Verification items for this drawing (mm, ordinates from the low corner). A direction names the side the tool comes from. Coordinates: 2 decimals unless noted, no trailing zeros. Order: outer loops, then holes, each group sorted by start corner. A loop starts at its lowest first (then second) coordinate and runs counter-clockwise, first axis right, second up. Notation, with made-up numbers: M 56,-11 L 113,-11 A31 ccw 113,17 Z; hole C 51,-9.75 d7. An arc over 180 degrees is marked long. One line per item, written item: value. Start each with the question number.
1) Sectioned sample at C-C, the plane y = 11.5. Enter the section's corners in (x, z).
2) Sectioned sample at D-D, the plane z = 6.5. Enter the section's corners in (x, y).
3) Sectioned sample at A-A, the plane x = 25. Enter the section's corners in (y, z).
4) Draft check along X on the marked faces 1, 2, 3 and 4. Enter one of: pulls with the +X half, pulls with the -X half, needs draft (parallel to the pull), parting line crosses it, or undercut.
5) Access from +Z, -Z, +X, -X, +Y, -Y to the whole of each face (thin tool, end or side, straight path). Record for the marked faces 5 and 6.
6) Sectioned sample at B-B, the plane z = 21.5. Enter the section's corners in (x, y).
7) Thickness scan on L1, parallel to X at y = 19, z = 24.5; L2, parallel to Y at x = 31, z = 13. Record the ranges inside material, lowest first. Write a range as from..to.
8) Go/stop test with flat-tipped pins: P1, Ø12, axis at x = 25, y = 7.5, coming from the +Z side; P2, Ø1.5, axis at x = 10.5, z = 22.5, coming from the +Y side; P3, Ø13, axis at y = 25, z = 21.5, coming from the -X side; P4, Ø3, axis at y = 23.5, z = 24.5, coming from the +X side. Record where each tip stops, or that it passes through.
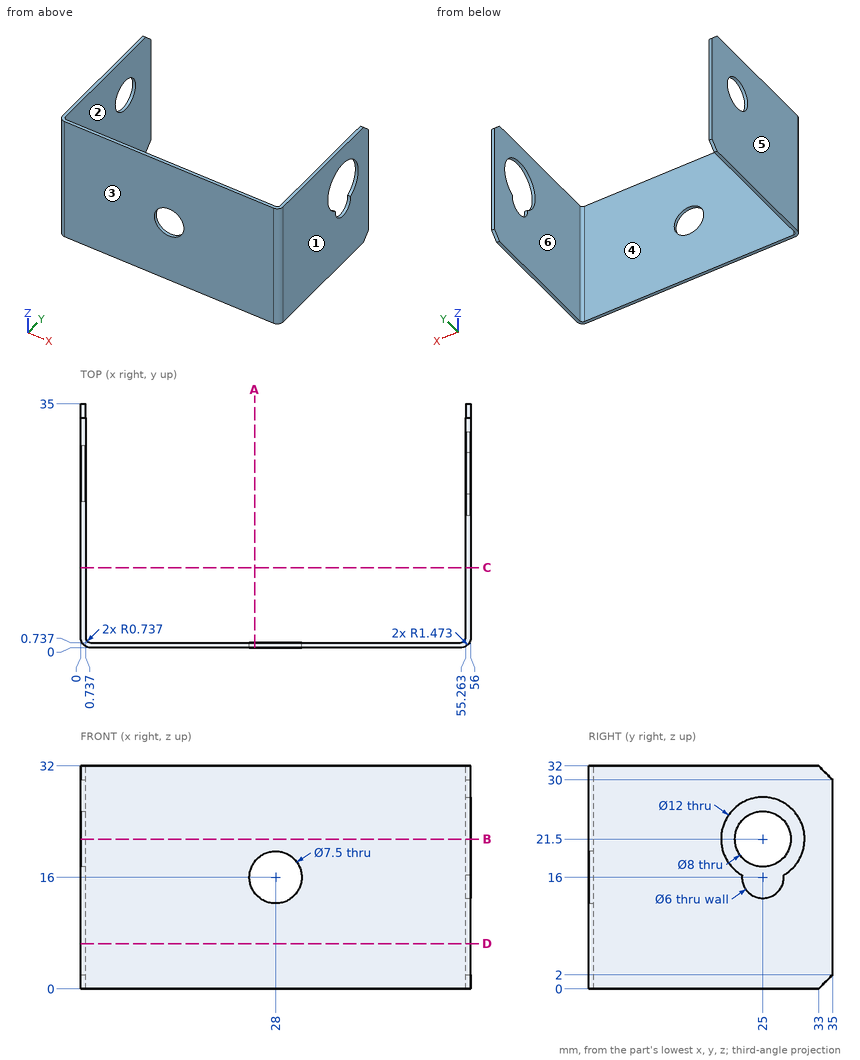
Final values:
1. outline: M 0,0 L 0.74,0 L 0.74,32 L 0,32 Z; M 55.26,0 L 56,0 L 56,32 L 55.26,32 Z
2. outline: M 0,1.47 A1.47 ccw 1.47,0 L 54.53,0 A1.47 ccw 56,1.47 L 56,35 L 55.26,35 L 55.26,1.47 A0.74 cw 54.53,0.74 L 1.47,0.74 A0.74 cw 0.74,1.47 L 0.74,35 L 0,35 Z
3. outline: M 0,0 L 0.74,0 L 0.74,13.75 L 0,13.75 Z; M 0,18.25 L 0.74,18.25 L 0.74,32 L 0,32 Z
4. face 1: pulls with the +X half
4. face 2: undercut
4. face 3: needs draft
4. face 4: undercut
5. face 5: +Z, -Z, -X, +Y, -Y
5. face 6: +Z, -Z, +Y
6. outline: M 0,1.47 A1.47 ccw 1.47,0 L 54.53,0 A1.47 ccw 56,1.47 L 56,19 L 55.26,19 L 55.26,1.47 A0.74 cw 54.53,0.74 L 1.47,0.74 A0.74 cw 0.74,1.47 L 0.74,21 L 0,21 Z; M 0,29 L 0.74,29 L 0.74,35 L 0,35 Z; M 55.26,31 L 56,31 L 56,35 L 55.26,35 Z
7. L1: x = 0..0.74, 55.26..56
7. L2: y = 0..0.74
8. P1: passes through
8. P2: stops at y = 0.74
8. P3: stops at x = 0
8. P4: stops at x = 0.74
